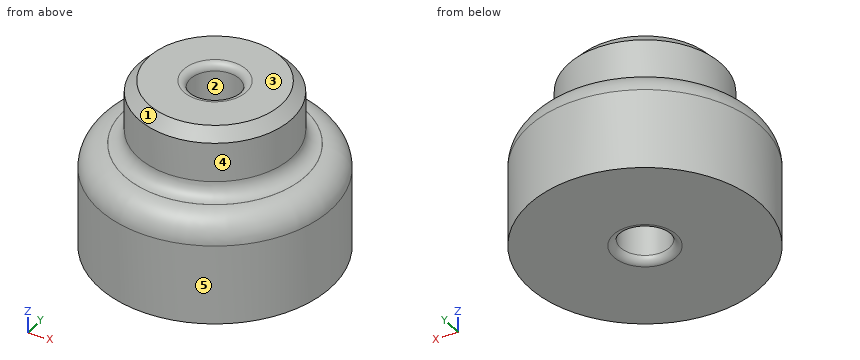
```python
from build123d import *


with BuildPart() as f1:
    # F0 (on Right) → F1 (revolve)
    with BuildSketch(Plane.YZ):
        with BuildLine():
            ThreePointArc((-1.143, 0), (-0.963395, 0.074395), (-0.889, 0.254))
            Line((-0.889, 0.254), (-0.889, 5.931143))
            ThreePointArc((-0.889, 5.931143), (-0.963395, 6.110748), (-1.143, 6.185143))
            Line((-1.143, 6.185143), (-2.412197, 6.185143))
            Line((-2.412197, 6.185143), (-2.794, 5.777119))
            Line((-2.794, 5.777119), (-2.794, 4.340756))
            ThreePointArc((-2.794, 4.340756), (-2.94279, 3.981545), (-3.302, 3.832756))
            Line((-3.302, 3.832756), (-3.30708, 3.832756))
            ThreePointArc((-3.30708, 3.832756), (-3.953658, 3.564934), (-4.22148, 2.918356))
            Line((-4.22148, 2.918356), (-4.22148, 0))
            Line((-4.22148, 0), (-1.143, 0))
        make_face()
    revolve(axis=Axis((0, 0, 3.175), (0, 0, 1)))


solid = f1.part
```
Model file for the job. Use its own axes, mm. Face numbers are marked on the shaded views. A direction names the side the tool comes from. Give positions to 0.01 mm unless a question says otherwise; leave off trailing zeros. Write each loop counter-clockwise with the first axis right and the second up, starting at its lowest first coordinate (ties: lowest second). Pieces come first, ordered by that corner, then holes. Notation, with made-up numbers: (75, 62.5) -> (79, 62.5) arc R31 ccw to (79, 86.5) -> close; hole circle Ø6 at (-21.5, 24). An arc over 180 degrees is marked (long way). Use CSV: the item, a comma, the result in double quotes. Start each with the question number.
1) Pin check, flat tips, straight feed: P1, Ø1.5, axis at y = -2.5, z = 2, coming from the -X side; P2, Ø2, axis at y = -3, z = 2, coming from the -X side. Stop position of each tip, or through.
2) Cut at C-C on z = 1. List the corners of the cut face in (x, y).
3) Cut at D-D on z = 3.5. List the corners of the cut face in (x, y), plus the area to 3 significant figures.
4) Tool access for the marked faces 4 and 5: list every direction of +Z, -Z, +X, -X, +Y, -Y with a clear straight run to the whole face (end or side of a thin tool).
5) Drill centre lines: L1, parallel to X at y = 0, z = 2.65; L2, parallel to X at y = 0, z = 3.4; L3, parallel to Y at x = 0.5, z = 3.75. Where is each one in solid material? Low to high.
6) Two-plate mould, pull along Y, no slides. Class the marked faces 1, 2 and 3: released by +Y, released by -Y, zero draft, split by the parting line, or undercut.
Final values:
1,P1,"stops at x = -3.84"
1,P2,"stops at x = -3.72"
2,outline,"circle Ø8.44 at (0, 0); hole circle Ø1.78 at (0, 0)"
3,outline,"circle Ø8.03 at (0, 0); hole circle Ø1.78 at (0, 0)"
3,area,"48.1 mm2"
4,face 4,"+Z"
4,face 5,"+Z, -Z"
5,L1,"x = -4.22 to -0.89, 0.89 to 4.22"
5,L2,"x = -4.08 to -0.89, 0.89 to 4.08"
5,L3,"y = -3.65 to -0.74, 0.74 to 3.65"
6,face 1,"split by the parting line"
6,face 2,"undercut"
6,face 3,"zero draft"
